from build123d import *

# Parameters (mm, degrees)
BOSS_EXTRUDE3_DEPTH = 1
SKETCH2_W           = 5
SKETCH2_H           = 30
CUT_EXTRUDE6_DEPTH  = 0.5
SKETCH3_R           = 5
CUT_EXTRUDE7_DEPTH  = 9


with BuildPart() as part:
    # Sketch1 → Boss-Extrude3 (new body)
    with BuildSketch(Plane.XY):
        Polygon((-24.880558789, 19.329851987), (-54.880558789, -7.127661123), (-54.880558789, -35.670148013), (-24.880558789, -35.670148013), align=None)
    extrude(amount=BOSS_EXTRUDE3_DEPTH)

    # Sketch2 → Cut-Extrude6 (cut)
    with BuildSketch(Plane.XY.offset(1)):
        with Locations((-27.380558789, 4.329851987)):
            Rectangle(SKETCH2_W, SKETCH2_H)
    extrude(amount=-CUT_EXTRUDE6_DEPTH, mode=Mode.SUBTRACT)

    # Sketch3 → Cut-Extrude7 (cut)
    with BuildSketch(Plane.XY.offset(1)):
        with Locations((-39.880558789, -27.670148013)):
            Circle(SKETCH3_R)
        with Locations((-39.880558789, -15.670148013)):
            Circle(SKETCH3_R)
    extrude(amount=-CUT_EXTRUDE7_DEPTH, mode=Mode.SUBTRACT)


solid = part.part
Geometry check sheet. Reference: the model listing, model coordinates, mm. Give positions to 0.01 mm unless a question says otherwise; leave off trailing zeros. Loops run counter-clockwise (first coordinate to the right, second up) from the corner with the lowest first, then second, coordinate; pieces in that order, holes last. Notation, with made-up numbers: M 22,24 L 30,24 A24 ccw 30,62 Z; hole C 87,48 d6. An arc over 180 degrees is marked long. Answer as a JSON object with one key per item and string values. Group by question number.
Item 1: Sectioned sample at B-B on y = -18. Record the boundary of the cut face in (x, z).
Item 2: Sectioned sample at C-C on z = 0.75. Record the boundary of the cut face in (x, y).
Item 3: Gauge pin test, flat ends, axial feed: pin 1 (4 mm diameter, centred on x = -27.5, y = 7, fed in from +Z); pin 2 (6 mm diameter, centred on x = -39.88, y = -15.67, fed in from +Z). Record the tip position at first contact, or that the pin passes through.
Item 4: Sectioned sample at D-D on y = -9. Record the boundary of the cut face in (x, z), plus the area to 3 significant figures.
Item 5: Mould release check, pull along X, two halves, no side actions. Record for faces 1 (the flat face through (-54.881, -21.2, 0.5)), 2 (the cylindrical face through (-43.566, -24.291, 0.507)), 3 (the flat face through (-27, 5, 0.5)): pulls with the +X half, pulls with the -X half, needs draft (parallel to the pull), parting line crosses it, or undercut.
Item 6: Sectioned sample at A-A on x = -44. Record the boundary of the cut face in (y, z).
Item 7: Material ranges on L1, parallel to Y at x = -39.75, z = 0.4; L2, parallel to Y at x = -43.75, z = 0.8; L3, parallel to Y at x = -28.75, z = 0.7, recorded low to high.
Findings below:
{
 "1": {"outline": "M -54.88,0 L -44.3,0 L -44.3,1 L -54.88,1 Z; M -35.46,0 L -24.88,0 L -24.88,1 L -35.46,1 Z"},
 "2": {"outline": "M -54.88,-35.67 L -24.88,-35.67 L -24.88,-10.67 L -29.88,-10.67 L -29.88,14.92 L -54.88,-7.13 Z; hole C -39.88,-27.67 d10; hole C -39.88,-15.67 d10"},
 "3": {"pin 1": "z = 0.5", "pin 2": "through"},
 "4": {"outline": "M -54.88,0 L -24.88,0 L -24.88,0.5 L -29.88,0.5 L -29.88,1 L -54.88,1 Z", "area": "27.5 mm2"},
 "5": {"face 1": "pulls with the -X half", "face 2": "undercut", "face 3": "needs draft"},
 "6": {"outline": "M -35.67,0 L -30.5,0 L -30.5,1 L -35.67,1 Z; M -24.84,0 L -18.5,0 L -18.5,1 L -24.84,1 Z; M -12.84,0 L 2.47,0 L 2.47,1 L -12.84,1 Z"},
 "7": {"L1": "-35.67 to -32.67, -22.67 to -20.67, -10.67 to 6.22", "L2": "-35.67 to -30.84, -24.5 to -18.84, -12.5 to 2.69", "L3": "-35.67 to -10.67"}
}
